Can you work these out from the model? Positions are in its coordinate system, mm. Round coordinates to 2 decimals unless told otherwise and drop trailing zeros. Loops run counter-clockwise (first coordinate to the right, second up) from the corner with the lowest first, then second, coordinate; pieces in that order, holes last. Notation, with made-up numbers: (6.25, 44) - (53.25, 44) arc R18 ccw to (53.25, 67) - close; hole circle Ø4 at (65, 10.25). An arc over 180 degrees is marked (long way). Answer as CSV lines item,"result".
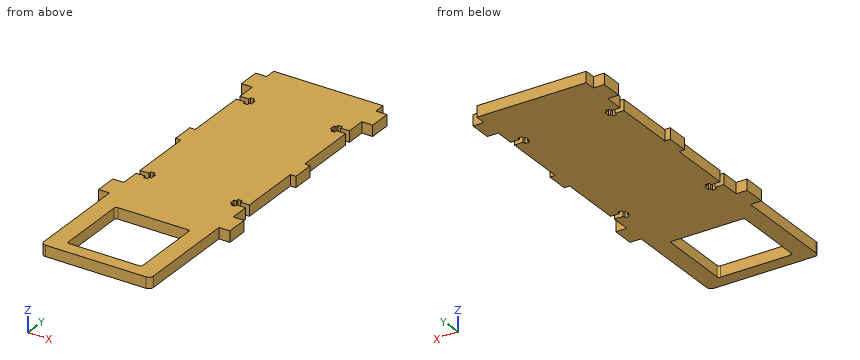
```python
from build123d import *

# Parameters (mm, degrees)
SKETCH1_W           = 63.5
SKETCH1_H           = 152.4
BOSS_EXTRUDE1_DEPTH = 6.35
SKETCH2_W           = 3.175
SKETCH2_H           = 12.7
SKETCH2_W_2         = 6.35
BOSS_EXTRUDE3_DEPTH = 6.35
SKETCH4_W           = 8.89
SKETCH4_H           = 3.302
SKETCH4_W_2         = 2.5
SKETCH4_H_2         = 6.5
CUT_EXTRUDE4_DEPTH  = 6.35
SKETCH5_W           = 63.5
SKETCH5_H           = 50.8
SKETCH5_W_2         = 43.18
SKETCH5_H_2         = 43.18
BOSS_EXTRUDE4_DEPTH = 6.35
SKETCH7_W           = 63.5
SKETCH7_H           = 3.81
BOSS_EXTRUDE5_DEPTH = 6.35
FILLET1_R           = 2.54
FILLET2_R           = 1.27


with BuildPart() as part:
    # Sketch1 → Boss-Extrude1 (new body)
    with BuildSketch(Plane.XY):
        with Locations((31.75, 76.2)):
            Rectangle(SKETCH1_W, SKETCH1_H)
    extrude(amount=BOSS_EXTRUDE1_DEPTH)

    # Sketch2 → Boss-Extrude3 (add)
    with BuildSketch(Plane.XY.offset(6.35)):
        with Locations((-1.5875, 76.2)):
            Rectangle(SKETCH2_W, SKETCH2_H)
        with Locations((66.675, 139.7)):
            Rectangle(SKETCH2_W_2, SKETCH2_H)
        with Locations((65.0875, 76.2)):
            Rectangle(SKETCH2_W, SKETCH2_H)
        with Locations((66.675, 12.7)):
            Rectangle(SKETCH2_W_2, SKETCH2_H)
        with Locations((-3.175, 12.7)):
            Rectangle(SKETCH2_W_2, SKETCH2_H)
        with Locations((-3.175, 139.7)):
            Rectangle(SKETCH2_W_2, SKETCH2_H)
    extrude(amount=-BOSS_EXTRUDE3_DEPTH)

    # Sketch4 → Cut-Extrude4 (cut)
    with BuildSketch(Plane.XY.offset(6.35)):
        with Locations((4.445, 120.65)):
            Rectangle(SKETCH4_W, SKETCH4_H)
        with Locations((6.37, 120.65)):
            Rectangle(SKETCH4_W_2, SKETCH4_H_2)
        with Locations((6.37, 31.75)):
            Rectangle(SKETCH4_W_2, SKETCH4_H_2)
        with Locations((4.445, 31.75)):
            Rectangle(SKETCH4_W, SKETCH4_H)
        with Locations((59.055, 31.75)):
            Rectangle(SKETCH4_W, SKETCH4_H)
        with Locations((57.13, 31.75)):
            Rectangle(SKETCH4_W_2, SKETCH4_H_2)
        with Locations((57.13, 120.65)):
            Rectangle(SKETCH4_W_2, SKETCH4_H_2)
        with Locations((59.055, 120.65)):
            Rectangle(SKETCH4_W, SKETCH4_H)
    extrude(amount=-CUT_EXTRUDE4_DEPTH, mode=Mode.SUBTRACT)

    # Sketch5 → Boss-Extrude4 (add)
    with BuildSketch(Plane.XY.offset(6.35)):
        with Locations((31.75, -25.4)):
            Rectangle(SKETCH5_W, SKETCH5_H)
        with Locations((31.75, -25.4)):
            Rectangle(SKETCH5_W_2, SKETCH5_H_2, mode=Mode.SUBTRACT)
    extrude(amount=-BOSS_EXTRUDE4_DEPTH)

    # Sketch7 → Boss-Extrude5 (add)
    with BuildSketch(Plane.XY.offset(6.35)):
        with Locations((31.75, -52.705)):
            Rectangle(SKETCH7_W, SKETCH7_H)
    extrude(amount=-BOSS_EXTRUDE5_DEPTH)

    # Fillet1
    fillet1_edges = [part.edges().sort_by_distance(p)[0] for p in [
        (63.5, -54.61, 3.175),
        (0, -54.61, 3.175),
    ]]
    fillet(fillet1_edges, radius=FILLET1_R)

    # Fillet2
    fillet2_edges = [part.edges().sort_by_distance(p)[0] for p in [
        (53.34, -46.99, 3.175),
        (10.16, -46.99, 3.175),
        (10.16, -3.81, 3.175),
        (53.34, -3.81, 3.175),
    ]]
    fillet(fillet2_edges, radius=FILLET2_R)


solid = part.part
```
Q1. I'm going to push flat-ended pins straight in: pin 1 Ø1.5 at (y, z) = (27, 4) entering from +X; pin 2 Ø1 at (y, z) = (32, 1.5) entering from -X; pin 3 Ø1.3 at (y, z) = (29.5, 3.5) entering from -X. Where does each tip first touch, or does it pass through?
Checks:
pin 1,"x = 63.5"
pin 2,"x = 8.89"
pin 3,"x = 0"
Q2. Imagine slicing it at C-C (y = 59.5). Write out the boundary of the cut face in (x, z).
Checks:
outline,"(0, 0) - (63.5, 0) - (63.5, 6.35) - (0, 6.35) - close"
Q3. Imagine slicing it at B-B (x = 21). Write out the boundary of the cut face in (y, z).
Checks:
outline,"(-54.61, 0) - (-46.99, 0) - (-46.99, 6.35) - (-54.61, 6.35) - close; (-3.81, 0) - (152.4, 0) - (152.4, 6.35) - (-3.81, 6.35) - close"
Q4. Imagine slicing it at A-A (y = -7.5). Write out the boundary of the cut face in (x, z).
Checks:
outline,"(0, 0) - (10.16, 0) - (10.16, 6.35) - (0, 6.35) - close; (53.34, 0) - (63.5, 0) - (63.5, 6.35) - (53.34, 6.35) - close"
Q5. If I drill on line 1 along Y through (x, z) = (-3, 2.75); line 2 along Y through (x, z) = (55.5, 1.5); line 3 along X through (y, z) = (-22.5, 3), over which ranges is the centre line in solid material (lowest first)? Write a range as [from, to].
Checks:
line 1,"[6.35, 19.05], [69.85, 82.55], [133.35, 146.05]"
line 2,"[-54.61, 30.1], [33.4, 119], [122.3, 152.4]"
line 3,"[0, 10.16], [53.34, 63.5]"
